Read the model definition and answer for the solid it produces. Units are mm, in the model's axes. Face numbers are marked on the shaded views. A direction names the side the tool comes from. Give positions to 0.01 mm unless a question says otherwise; leave off trailing zeros. Loops run counter-clockwise (first coordinate to the right, second up) from the corner with the lowest first, then second, coordinate; pieces in that order, holes last. Notation, with made-up numbers: (76, 23) - (105, 23) arc R9 cw to (105, 39) - close; hole circle Ø9 at (-2.5, 83). An arc over 180 degrees is marked (long way). Write each question's results on one line, items separated by ' | '. Start each with the question number.
Q1. The part is cut by section A-A, the plane x = 0. Write down the section's boundary in (y, z).
Q2. Find the intervals of material crossed by line 1 (Z direction, x = 26.5, y = 33); line 2 (Z direction, x = -28, y = 33); line 3 (Y direction, x = -33, z = 8), in increasing order. Write a range as from..to.
Q3. The part is cut by section D-D, the plane y = 102. Write down the section's boundary in (x, z).
Q4. Determine the mould class of the marked faces 1, 2 and 3 for opening direction Z: +Z half, -Z half, draft (parallel to the pull), parting line (faces both ways), or undercut.
Q5. The part is cut by section C-C, the plane y = 33. Write down the section's boundary in (x, z), plus the area to 3 significant figures.
Q6. Given pin 1 (7 mm diameter, centred on y = 31, z = 3, fed in from +X); pin 2 (12 mm diameter, centred on x = 9.5, y = 107, fed in from +Z); pin 3 (2 mm diameter, centred on x = 17.5, y = 47, fed in from -Z), each flat-ended and moving along its own axis, determine where each tip first touches the part or whether it passes through.
Q7. For the marked faces 4, 5 and 6, determine the directions among +Z, -Z, +X, -X, +Y, -Y from which every point of the face is accessible in a straight line to the end or side of a thin tool.
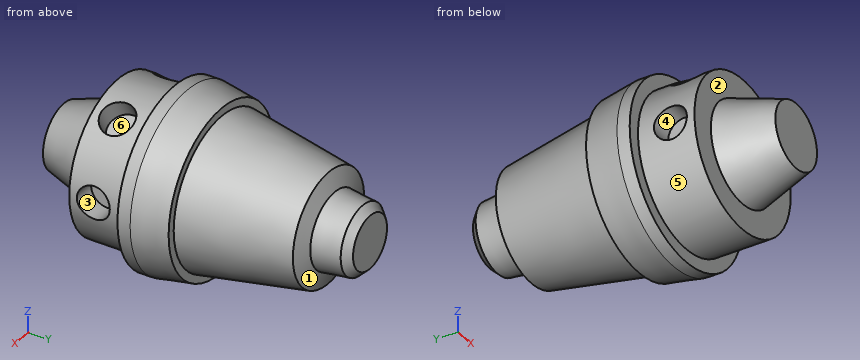
```python
from build123d import *

# Parameters (mm, degrees)
SKETCH_2_R          = 7
CUT_EXTRUDE_1_DEPTH = 15
SKETCH_3_R          = 7
CUT_EXTRUDE_2_DEPTH = 15
SKETCH_4_R          = 7
CUT_EXTRUDE_3_DEPTH = 15
SKETCH_5_R          = 7
CUT_EXTRUDE_4_DEPTH = 15


with BuildPart() as part:
    # Эскиз1 → Повернуть1 (revolve)
    with BuildSketch(Plane.XY):
        Polygon((0, 0), (13.832956578, 0), (21.093288223, 22.779290537), (32, 22.779290537), (32, 46.779290537), (37.5, 46.779290537), (37.5, 52.174655371), (35, 66.934934907), (31.630138236, 66.934934907), (23.700917658, 112.523953152), (15.988556841, 114.982076121), (14.50917162, 126.947847272), (11.301374522, 130.155644371), (0, 130.155644371), align=None)
    revolve(axis=Axis((0, 138.703973398, 0), (0, -1, 0)))

    # Эскиз2 → Вырез-Вытянуть1 (cut)
    with BuildSketch(Plane(origin=(-37.5, 0, 0), x_dir=(0, 1, 0), z_dir=(-1, 0, 0))):
        with Locations((33, 0)):
            Circle(SKETCH_2_R)
    extrude(amount=-CUT_EXTRUDE_1_DEPTH, mode=Mode.SUBTRACT)

    # Эскиз3 → Вырез-Вытянуть2 (cut)
    with BuildSketch(Plane(origin=(18.75, 0, 32.475952642), x_dir=(0, 1, 0), z_dir=(0.5, 0, 0.866025404))):
        with Locations((33, 0)):
            Circle(SKETCH_3_R)
    extrude(amount=-CUT_EXTRUDE_2_DEPTH, mode=Mode.SUBTRACT)

    # Эскиз4 → Вырез-Вытянуть3 (cut)
    with BuildSketch(Plane(origin=(-23.087305325, 0, 29.55040326), x_dir=(0, 1, 0), z_dir=(-0.615661475, 0, 0.788010754))):
        with Locations((33, 0)):
            Circle(SKETCH_4_R)
    extrude(amount=-CUT_EXTRUDE_3_DEPTH, mode=Mode.SUBTRACT)

    # Эскиз5 → Вырез-Вытянуть4 (cut)
    with BuildSketch(Plane.YZ.offset(37.5)):
        with Locations((33, 0)):
            Circle(SKETCH_5_R)
    extrude(amount=-CUT_EXTRUDE_4_DEPTH, mode=Mode.SUBTRACT)


solid = part.part
```
Check sheet entries:
1) outline: (0, -13.83) - (22.78, -21.09) - (22.78, -32) - (46.78, -32) - (46.78, -37.5) - (52.17, -37.5) - (66.93, -35) - (66.93, -31.63) - (112.52, -23.7) - (114.98, -15.99) - (126.95, -14.51) - (130.16, -11.3) - (130.16, 11.3) - (126.95, 14.51) - (114.98, 15.99) - (112.52, 23.7) - (66.93, 31.63) - (66.93, 35) - (52.17, 37.5) - (46.78, 37.5) - (46.78, 32) - (22.78, 32) - (22.78, 21.09) - (0, 13.83) - close
2) line 1: z = -17.94..-7, 7..17.94 | line 2: z = -15.49..-7, 7..15.49 | line 3: y = 46.78..66.93
3) outline: circle Ø51.06 at (0, 0)
4) face 1: parting line | face 2: draft | face 3: undercut
5) outline: (-31.22, -7) arc R32 ccw to (31.22, -7) - (22.5, -7) - (22.5, 7) - (31.22, 7) arc R32 ccw to (21.67, 23.54) - (17.31, 15.99) - (5.19, 22.99) - (9.55, 30.54) arc R32 ccw to (-13.71, 28.92) - (-8.34, 22.04) - (-19.37, 13.42) - (-24.74, 20.3) arc R32 ccw to (-31.22, 7) - (-22.5, 7) - (-22.5, -7) - close | area: 2,700 mm^2
6) pin 1: stops at x = 31.59 | pin 2: stops at z = 24.85 | pin 3: stops at z = -33.67
7) face 4: -X | face 5: -Y | face 6: none
